Model file for the job. Use its own axes, mm. A direction names the side the tool comes from. Coordinates: 2 decimals unless noted, no trailing zeros. Order: outer loops, then holes, each group sorted by start corner. A loop starts at its lowest first (then second) coordinate and runs counter-clockwise, first axis right, second up. Notation, with made-up numbers: (31, 48.25) -> (85, 48.25) arc R15 ccw to (85, 71.25) -> close; hole circle Ø1 at (-21.75, -31.75). An arc over 180 degrees is marked (long way). Use CSV: the item, a comma, the result in double quotes. Start each with the question number.
(1) Pin check, flat tips, straight feed: pin 1 Ø3 at (x, z) = (66.7, -8.8) entering from +Y; pin 2 Ø3 at (x, z) = (36, -8.8) entering from -Y. Stop position of each tip, or through.
(2) Tool access for faces 4 (the cylindrical face through (83.846, 2.218, -24.325)), 5 (the flat face through (23, 1.5, -7)): list every direction of +Z, -Z, +X, -X, +Y, -Y with a clear straight run to the whole face (end or side of a thin tool).
(3) Pull direction X, two halves, no side cores. Call faces 1 (the flat face through (0, 2, -24)), 2 (the cylindrical face through (46.05, 1.726, -36.188)), 3 (the flat face through (45, 2, 0)): pulls with the +X half, pulls with the -X half, needs draft (parallel to the pull), parting line crosses it, or undercut.
(4) Cut at B-B on y = 2.5. Give the number of separate pieces and of enclosed holes in the cut face, plus the area to 3 significant figures.
(5) Cut at A-A on x = 28.5. Write the cut outline in (y, z), plus the area to 3 significant figures.
(6) Probe L1, parallel to X at y = 0.85, z = -8.8; L2, parallel to X at y = 3.2, z = -21; L3, parallel to X at y = 1.8, z = -10.5. List the from-to ranges inside material, lowest first.
(7) Cut at C-C on z = -44.5. Write the cut outline in (x, y), plus the area to 3 significant figures.
```python
from build123d import *

# Parameters (mm, degrees)
SKETCH1_W           = 90.71
SKETCH1_H           = 47.8
SKETCH1_R           = 1.5
SKETCH1_R_2         = 1.25
SKETCH1_R_3         = 12.5
BOSS_EXTRUDE1_DEPTH = 4.5
SKETCH2_R           = 3.5
CUT_EXTRUDE1_DEPTH  = 3
CHAMFER1_SIZE       = 1
FILLET1_R           = 1


with BuildPart() as part:
    # Sketch1 → Boss-Extrude1 (new body)
    with BuildSketch(Plane(origin=(0, 0, 0), x_dir=(1, 0, 0), z_dir=(0, 1, 0))):
        with Locations((45.355, 23.9)):
            Rectangle(SKETCH1_W, SKETCH1_H)
        with Locations(Location((85.01, 4.6, 0), (0, 0, 270))):
            Circle(SKETCH1_R, mode=Mode.SUBTRACT)
        with Locations(Location((85.31, 24, 0), (0, 0, 270))):
            Circle(SKETCH1_R, mode=Mode.SUBTRACT)
        with Locations(Location((84.91, 44.12, 0), (0, 0, 270))):
            Circle(SKETCH1_R, mode=Mode.SUBTRACT)
        with Locations(Location((5.8, 44.12, 0), (0, 0, 270))):
            Circle(SKETCH1_R, mode=Mode.SUBTRACT)
        with Locations(Location((5.4, 24, 0), (0, 0, 270))):
            Circle(SKETCH1_R, mode=Mode.SUBTRACT)
        with Locations(Location((5.7, 4.6, 0), (0, 0, 270))):
            Circle(SKETCH1_R, mode=Mode.SUBTRACT)
        with Locations(Location((28.5, 21.7, 0), (0, 0, 270))):
            Circle(SKETCH1_R_2, mode=Mode.SUBTRACT)
        with Locations(Location((22.8, 8.8, 0), (0, 0, 270))):
            Circle(SKETCH1_R_2, mode=Mode.SUBTRACT)
        with Locations(Location((36, 8.8, 0), (0, 0, 270))):
            Circle(SKETCH1_R_2, mode=Mode.SUBTRACT)
        with Locations(Location((54.1, 8.8, 0), (0, 0, 270))):
            Circle(SKETCH1_R_2, mode=Mode.SUBTRACT)
        with Locations(Location((66.7, 8.8, 0), (0, 0, 270))):
            Circle(SKETCH1_R_2, mode=Mode.SUBTRACT)
        with Locations(Location((62.5, 21.7, 0), (0, 0, 270))):
            Circle(SKETCH1_R_2, mode=Mode.SUBTRACT)
        with Locations(Location((45.5, 23.7, 0), (0, 0, 270))):
            Circle(SKETCH1_R_3, mode=Mode.SUBTRACT)
    extrude(amount=BOSS_EXTRUDE1_DEPTH)

    # Sketch2 → Cut-Extrude1 (cut)
    with BuildSketch(Plane(origin=(0, 4.5, 0), x_dir=(1, 0, 0), z_dir=(0, 1, 0))):
        with Locations(Location((28.5, 21.7, 0), (0, 0, 270))):
            Circle(SKETCH2_R)
        with Locations(Location((22.8, 8.8, 0), (0, 0, 270))):
            Circle(SKETCH2_R)
        with Locations(Location((36, 8.8, 0), (0, 0, 270))):
            Circle(SKETCH2_R)
        with Locations(Location((54.1, 8.8, 0), (0, 0, 270))):
            Circle(SKETCH2_R)
        with Locations(Location((66.7, 8.8, 0), (0, 0, 270))):
            Circle(SKETCH2_R)
        with Locations(Location((62.5, 21.7, 0), (0, 0, 270))):
            Circle(SKETCH2_R)
    extrude(amount=-CUT_EXTRUDE1_DEPTH, mode=Mode.SUBTRACT)

    # Chamfer1
    chamfer1_edges = [part.edges().sort_by_distance(p)[0] for p in [
        (45.5, 4.5, -36.2),
    ]]
    chamfer(chamfer1_edges, length=CHAMFER1_SIZE)

    # Fillet1
    fillet1_edges = [part.edges().sort_by_distance(p)[0] for p in [
        (90.71, 4.5, -23.9),
        (45.355, 4.5, -47.8),
        (0, 4.5, -23.9),
        (45.355, 0, -47.8),
        (90.71, 0, -23.9),
        (45.355, 0, 0),
        (0, 0, -23.9),
        (0, 2.25, -47.8),
        (90.71, 2.25, -47.8),
        (90.71, 2.25, 0),
        (0, 2.25, 0),
        (45.355, 4.5, 0),
    ]]
    fillet(fillet1_edges, radius=FILLET1_R)


solid = part.part
```
Outcome:
1,pin 1,"y = 1.5"
1,pin 2,"y = 0"
2,face 4,"+Y, -Y"
2,face 5,"+Y"
3,face 1,"pulls with the -X half"
3,face 2,"undercut"
3,face 3,"needs draft"
4,separate pieces,"1"
4,enclosed holes,"13"
4,area,"3,570 mm2"
5,outline,"(0, -46.8) arc R1 ccw to (1, -47.8) -> (3.5, -47.8) arc R1 ccw to (4.5, -46.8) -> (4.5, -25.2) -> (1.5, -25.2) -> (1.5, -22.95) -> (0, -22.95) -> close; (0, -20.45) -> (1.5, -20.45) -> (1.5, -18.2) -> (4.5, -18.2) -> (4.5, -1) arc R1 ccw to (3.5, 0) -> (1, 0) arc R1 ccw to (0, -1) -> close"
5,area,"189 mm2"
6,L1,"0.01 to 21.55, 24.05 to 34.75, 37.25 to 52.85, 55.35 to 65.45, 67.95 to 90.7"
6,L2,"0 to 25.07, 31.93 to 33.3, 57.7 to 59.07, 65.93 to 90.71"
6,L3,"0 to 19.74, 25.86 to 32.94, 39.06 to 51.04, 57.16 to 63.64, 69.76 to 90.71"
7,outline,"(0, 1) arc R1 ccw to (1, 0) -> (4.35, 0) -> (4.35, 4.5) -> (1, 4.5) arc R1 ccw to (0, 3.5) -> close; (7.25, 0) -> (83.46, 0) -> (83.46, 4.5) -> (7.25, 4.5) -> close; (86.36, 0) -> (89.71, 0) arc R1 ccw to (90.71, 1) -> (90.71, 3.5) arc R1 ccw to (89.71, 4.5) -> (86.36, 4.5) -> close"
7,area,"381 mm2"
